```python
from build123d import *

# Parameters (mm, degrees)
F1_DEPTH = 45
F3_R     = 2.5
F4_DEPTH = 2


with BuildPart() as f1:
    # F0 (on Right) → F1 (new body, symmetric)
    with BuildSketch(Plane.YZ):
        Polygon((0, -29), (0, 0), (-43.5, 0), (-43.5, -2), (-2, -2), (-2, -27), (-43.5, -27), (-43.5, -29), align=None)
    extrude(amount=F1_DEPTH, both=True)

    # F2: F1 across plane


with BuildPart() as f1_1:
    add(f1.part)
    add(f1.part.mirror(Plane.XZ))

    # F3 (on face) → F4 (cut, through all)
    with BuildSketch(Plane.XY):
        with Locations((35, 31)):
            Circle(F3_R)
        with Locations((0, 31)):
            Circle(F3_R)
        with Locations((-35, 31)):
            Circle(F3_R)
        with Locations((-35, -31)):
            Circle(F3_R)
        with Locations((0, -31)):
            Circle(F3_R)
        with Locations((35, -31)):
            Circle(F3_R)
    extrude(amount=-F4_DEPTH, mode=Mode.SUBTRACT)


solid = f1_1.part
```
Could you check a few things on this model? Use its own coordinates, in mm. A direction names the side the tool comes from. Coordinates: 2 decimals unless noted, no trailing zeros. Order: outer loops, then holes, each group sorted by start corner. A loop starts at its lowest first (then second) coordinate and runs counter-clockwise, first axis right, second up. Notation, with made-up numbers: M 46,85 L 90,85 A30 cw 90,110 Z; hole C -32,4.25 d9. An arc over 180 degrees is marked long. Use a Markdown table: item, result. Add a question column.
Q1. Which directions (+Z, -Z, +X, -X, +Y, -Y) give clear straight access to the entire face, cutting with the end or side of a thin tool? Please do faces 1 (the flat face through (1, 22, -27)), 2 (the flat face through (1, -22, -27)), 3 (the cylindrical face through (36.34, 33.11, -0.99)).
Q2. I want a section at C-C on x = 4. List the corners of the cut face in (y, z) for me, then the cut area to 3 significant figures.
Q3. I want a section at D-D on y = 31. List the corners of the cut face in (x, z) for me, then the cut area to 3 significant figures.
Q4. I'm going to push flat-ended pins straight in: pin 1 (3 mm diameter, centred on x = 0, y = -31, fed in from +Z); pin 2 (10 mm diameter, centred on x = -28, z = -18.5, fed in from -Y); pin 3 (8 mm diameter, centred on x = 19.5, z = -13.5, fed in from +Y). Where does each tip first touch, or does it pass through?
Q5. We'd pull the mould along Z, two halves only. Please class faces 4 (the flat face through (1, -1, 0)), 5 (the flat face through (1, 23, -2)), 6 (the flat face through (1, -43.5, -28)): pulls with the +Z half, pulls with the -Z half, needs draft (parallel to the pull), parting line crosses it, or undercut.
Q6. If I drill on L1, parallel to Y at x = 0, z = -1.55; L2, parallel to Z at x = 9.5, y = -9.5; L3, parallel to Y at x = 25, z = -21.25, over which ranges is the centre line in solid material (lowest first)?
Q7. I want a section at A-A on y = 10. List the corners of the cut face in (x, z) for me.
Q8. I want a section at B-B on x = -35. List the corners of the cut face in (y, z) for me.
Checked values:
| question | item | result |
|---|---|---|
| 1 | face 1 | +X, -X, +Y |
| 1 | face 2 | +X, -X, -Y |
| 1 | face 3 | +Z |
| 2 | outline | M -43.5,-29 L 43.5,-29 L 43.5,-27 L 2,-27 L 2,-2 L 43.5,-2 L 43.5,0 L -43.5,0 L -43.5,-2 L -2,-2 L -2,-27 L -43.5,-27 Z |
| 2 | area | 448 mm² |
| 3 | outline | M -45,-29 L 45,-29 L 45,-27 L -45,-27 Z; M -45,-2 L -37.5,-2 L -37.5,0 L -45,0 Z; M -32.5,-2 L -2.5,-2 L -2.5,0 L -32.5,0 Z; M 2.5,-2 L 32.5,-2 L 32.5,0 L 2.5,0 Z; M 37.5,-2 L 45,-2 L 45,0 L 37.5,0 Z |
| 3 | area | 330 mm² |
| 4 | pin 1 | z = -27 |
| 4 | pin 2 | y = -2 |
| 4 | pin 3 | y = 2 |
| 5 | face 4 | pulls with the +Z half |
| 5 | face 5 | undercut |
| 5 | face 6 | needs draft |
| 6 | L1 | -43.5 to -33.5, -28.5 to 28.5, 33.5 to 43.5 |
| 6 | L2 | -29 to -27, -2 to 0 |
| 6 | L3 | -2 to 2 |
| 7 | outline | M -45,-29 L 45,-29 L 45,-27 L -45,-27 Z; M -45,-2 L 45,-2 L 45,0 L -45,0 Z |
| 8 | outline | M -43.5,-29 L 43.5,-29 L 43.5,-27 L 2,-27 L 2,-2 L 28.5,-2 L 28.5,0 L -28.5,0 L -28.5,-2 L -2,-2 L -2,-27 L -43.5,-27 Z; M -43.5,-2 L -33.5,-2 L -33.5,0 L -43.5,0 Z; M 33.5,-2 L 43.5,-2 L 43.5,0 L 33.5,0 Z |
